```python
from build123d import *

# Parameters (mm, degrees)
SCHIZZO1_R                   = 13
ESTRUSIONE_ESTRUSIONE1_DEPTH = 7
SCHIZZO2_R                   = 17
SCHIZZO2_R_2                 = 13
ESTRUSIONE_ESTRUSIONE2_DEPTH = 8
SMUSSO1_SIZE                 = 0.25
SMUSSO2_SIZE                 = 0.25
RACCORDO1_R                  = 0.25
RACCORDO2_R                  = 0.25
SCHIZZO3_R                   = 2.25
TAGLIO_ESTRUSIONE1_DEPTH     = 34.271609519
SCHIZZO4_R                   = 4
TAGLIO_ESTRUSIONE2_DEPTH     = 4
RIPETIZIONECIRCOLARE1_COUNT  = 4
SMUSSO3_SIZE                 = 0.1


with BuildPart() as part:
    # Schizzo1 → Estrusione-Estrusione1 (new body)
    with BuildSketch(Plane.XY):
        Polygon((-21, 15.769552622), (-15.769552622, 21), (15.769552622, 21), (21, 15.769552622), (21, -15.769552622), (15.769552622, -21), (-15.769552622, -21), (-21, -15.769552622), align=None)
        Circle(SCHIZZO1_R, mode=Mode.SUBTRACT)
    extrude(amount=ESTRUSIONE_ESTRUSIONE1_DEPTH)

    # Schizzo2 → Estrusione-Estrusione2 (add)
    with BuildSketch(Plane.XY.offset(7)):
        with Locations(Location((0, 0, 0), (0, 0, 180))):
            Circle(SCHIZZO2_R)
        Circle(SCHIZZO2_R_2, mode=Mode.SUBTRACT)
    extrude(amount=ESTRUSIONE_ESTRUSIONE2_DEPTH)

    # Smusso1
    smusso1_edges = [part.edges().sort_by_distance(p)[0] for p in [
        (0, 21, 0),
        (18.384776311, 18.384776311, 0),
        (-13, 0, 0),
        (21, 0, 0),
        (18.384776311, -18.384776311, 0),
        (0, -21, 0),
        (-18.384776311, -18.384776311, 0),
        (-21, 0, 0),
        (-18.384776311, 18.384776311, 0),
    ]]
    chamfer(smusso1_edges, length=SMUSSO1_SIZE)

    # Smusso2
    smusso2_edges = [part.edges().sort_by_distance(p)[0] for p in [
        (17, 0, 15),
        (-13, 0, 15),
    ]]
    chamfer(smusso2_edges, length=SMUSSO2_SIZE)

    # Raccordo1
    raccordo1_edges = [part.edges().sort_by_distance(p)[0] for p in [
        (17, 0, 7),
    ]]
    fillet(raccordo1_edges, radius=RACCORDO1_R)

    # Raccordo2
    raccordo2_edges = [part.edges().sort_by_distance(p)[0] for p in [
        (-18.384776311, 18.384776311, 7),
        (-21, 0, 7),
        (-18.384776311, -18.384776311, 7),
        (0, -21, 7),
        (18.384776311, -18.384776311, 7),
        (21, 0, 7),
        (18.384776311, 18.384776311, 7),
        (0, 21, 7),
    ]]
    fillet(raccordo2_edges, radius=RACCORDO2_R)

    # Schizzo3 → Taglio-Estrusione1 (cut, through all)
    with BuildSketch(Plane(origin=(0, 0, 0), x_dir=(-1, 0, 0), z_dir=(0, 0, -1))):
        with Locations((-14.849242405, 14.849242405)):
            Circle(SCHIZZO3_R)
    taglio_estrusione1 = extrude(amount=-TAGLIO_ESTRUSIONE1_DEPTH, mode=Mode.SUBTRACT)

    # Schizzo4 → Taglio-Estrusione2 (cut)
    with BuildSketch(Plane(origin=(0, 0, 0), x_dir=(-1, 0, 0), z_dir=(0, 0, -1))):
        with Locations((-14.849242405, 14.849242405)):
            Circle(SCHIZZO4_R)
    taglio_estrusione2 = extrude(amount=-TAGLIO_ESTRUSIONE2_DEPTH, mode=Mode.SUBTRACT)

    # RipetizioneCircolare1: Taglio-Estrusione1, Taglio-Estrusione2 ×4 about axis
    ripetizionecircolare1_axis = Axis((0, 0, 0), (0, 0, 1))
    add([taglio_estrusione1.rotate(ripetizionecircolare1_axis, i * 360 / RIPETIZIONECIRCOLARE1_COUNT) for i in range(1, RIPETIZIONECIRCOLARE1_COUNT)], mode=Mode.SUBTRACT)
    add([taglio_estrusione2.rotate(ripetizionecircolare1_axis, i * 360 / RIPETIZIONECIRCOLARE1_COUNT) for i in range(1, RIPETIZIONECIRCOLARE1_COUNT)], mode=Mode.SUBTRACT)

    # Smusso3
    smusso3_edges = [part.edges().sort_by_distance(p)[0] for p in [
        (18.849242405, 14.849242405, 0),
        (14.849242405, -17.099242405, 7),
        (-17.099242405, -14.849242405, 7),
        (-14.849242405, 17.099242405, 7),
        (14.849242405, -18.849242405, 0),
        (-18.849242405, -14.849242405, 0),
        (-14.849242405, 18.849242405, 0),
        (17.099242405, 14.849242405, 7),
    ]]
    chamfer(smusso3_edges, length=SMUSSO3_SIZE)


solid = part.part
```
The listing builds one solid part. Answer for the finished solid, in the listing's coordinates (mm). A direction names the side the tool comes from. Give positions to 0.01 mm unless a question says otherwise; leave off trailing zeros. Write each loop counter-clockwise with the first axis right and the second up, starting at its lowest first coordinate (ties: lowest second). Pieces come first, ordered by that corner, then holes. Notation, with made-up numbers: (-19, 85.5) -> (20, 85.5) arc R8 cw to (20, 90.5) -> close; hole circle Ø8 at (30, 40.25). An arc over 180 degrees is marked (long way). Write item = value, one per line. Start each with the question number.
1) The part is cut by section C-C, the plane z = 2. Determine the outline of the cut face in (x, y), and give its area (3 significant figures).
2) Each of these flat-tipped pins is pushed along its axis until it touches: pin 1 (10.5 mm diameter, centred on x = 14.85, y = -14.85, fed in from -Z); pin 2 (5 mm diameter, centred on x = 14.85, y = 14.85, fed in from -Z); pin 3 (7 mm diameter, centred on x = -14.85, y = -14.85, fed in from +Z); pin 4 (1.5 mm diameter, centred on y = 9.5, z = 11.5, fed in from -X). Where does it stop, or does it pass through?
3) Determine the mould class of faces 4 (the face through (18.4, 18.3, 6.9)), 5 (the face through (-13, 13, 4)), 6 (the face through (10, 10, 0)) for opening direction X: +X half, -X half, draft (parallel to the pull), parting line (faces both ways), or undercut.
4) Straight lines are drawn through the part: line 1 along Y through (x, z) = (-15, 5); line 2 along Y through (x, z) = (0, 11). For each, find the intervals that lie inside material, in ascending order.
5) The part is cut by section D-D, the plane z = 13. Determine the outline of the cut face in (x, y), and give its area (3 significant figures).
6) The part is cut by section A-A, the plane x = 0. Determine the outline of the cut face in (y, z), and give its area (3 significant figures).
7) Which of the six approach directions +Z, -Z, +X, -X, +Y, -Y give full straight-line access (tool end or side, diameter ignored) to faces 1 (the face through (-17.55, 17.8, 2.02)), 2 (the face through (2.213, -16.855, 10.948)), 3 (the face through (-18.35, -18.42, 3.45))?
Solutions:
q1.outline = (-21, -15.77) -> (-15.77, -21) -> (15.77, -21) -> (21, -15.77) -> (21, 15.77) -> (15.77, 21) -> (-15.77, 21) -> (-21, 15.77) -> close; hole circle Ø8 at (-14.85, -14.85); hole circle Ø8 at (-14.85, 14.85); hole circle Ø26 at (0, 0); hole circle Ø8 at (14.85, -14.85); hole circle Ø8 at (14.85, 14.85)
q1.area = 977 mm²
q2.pin_1 = 0
q2.pin_2 = 4
q2.pin_3 = 7
q2.pin_4 = -14.58
q3.face_4 = +X half
q3.face_5 = undercut
q3.face_6 = draft
q4.line_1 = -21 to -17.09, -12.6 to 12.6, 17.09 to 21
q4.line_2 = -17 to -13, 13 to 17
q5.outline = circle Ø34 at (0, 0); hole circle Ø26 at (0, 0)
q5.area = 377 mm²
q6.outline = (-21, 0.25) -> (-20.75, 0) -> (-13.25, 0) -> (-13, 0.25) -> (-13, 14.75) -> (-13.25, 15) -> (-16.75, 15) -> (-17, 14.75) -> (-17, 7.25) arc R0.25 cw to (-17.25, 7) -> (-20.75, 7) arc R0.25 ccw to (-21, 6.75) -> close; (13, 0.25) -> (13.25, 0) -> (20.75, 0) -> (21, 0.25) -> (21, 6.75) arc R0.25 ccw to (20.75, 7) -> (17.25, 7) arc R0.25 cw to (17, 7.25) -> (17, 14.75) -> (16.75, 15) -> (13.25, 15) -> (13, 14.75) -> close
q6.area = 176 mm²
q7.face_1 = -Z
q7.face_2 = +Z
q7.face_3 = +Z, -Z, -X, -Y
